Autodesk Inventor part; units mm, degrees
ref_plane "YZ Plane" through (0, 0, 0) normal (1, 0, 0) x (0, 1, 0)
ref_plane "XZ Plane" through (0, 0, 0) normal (0, 1, 0) x (-1, 0, 0)
ref_plane "XY Plane" through (0, 0, 0) normal (0, 0, 1) x (1, 0, 0)
sketch "Sketch1" plane through (0, 0, 0) normal (0, 1, 0) x (-1, 0, 0)
  line L0 (-690, -330) -> (690, -330)
  line L1 (690, -330) -> (690, 330)
  line L2 (690, 330) -> (-690, 330)
  line L3 (-690, 330) -> (-690, -330)
  line L4 (-690, -330) -> (690, 330) construction
  line L5 (690, -330) -> (-690, 330) construction
  point P0 (0, 0)
  dimension "d0" = 1380
  dimension "d1" = 660
extrude "Extrusion1" add sketch "Sketch1" along normal blind 60
sketch "Sketch2" plane through (0, 60, 0) normal (0, 1, 0) x (1, 0, 0)
  line L0 (-660, 300) -> (-360, 300) construction
  line L1 (-360, 300) -> (-360, -300) construction
  line L2 (-360, -300) -> (-660, -300) construction
  line L3 (-660, -300) -> (-660, 300) construction
  line L4 (-660, 300) -> (-360, -300) construction
  line L5 (-360, 300) -> (-660, -300) construction
  line L6 (-690, 330) -> (-690, -330)
  line L7 (-690, 0) -> (690, 0) construction
  line L8 (690, -330) -> (690, 330) construction
  line L9 (-370, 290) -> (-650, 290)
  line L10 (-650, 290) -> (-650, -290)
  line L11 (-650, -290) -> (-370, -290)
  line L12 (-370, -290) -> (-370, 290)
  line L13 (-20, 300) -> (-20, -300) construction
  line L14 (-30, -290) -> (-30, 290)
  line L15 (-30, 290) -> (-310, 290)
  line L16 (-320, 300) -> (-20, 300) construction
  line L17 (-310, 290) -> (-310, -290)
  line L18 (-320, -300) -> (-320, 300) construction
  line L19 (-320, 300) -> (-20, -300) construction
  line L20 (-20, 300) -> (-320, -300) construction
  line L21 (-310, -290) -> (-30, -290)
  line L22 (-20, -300) -> (-320, -300) construction
  line L23 (320, 300) -> (320, -300) construction
  line L24 (310, -290) -> (310, 290)
  line L25 (310, 290) -> (30, 290)
  line L26 (20, 300) -> (320, 300) construction
  line L27 (30, 290) -> (30, -290)
  line L28 (20, -300) -> (20, 300) construction
  line L29 (20, 300) -> (320, -300) construction
  line L30 (320, 300) -> (20, -300) construction
  line L31 (30, -290) -> (310, -290)
  line L32 (320, -300) -> (20, -300) construction
  line L33 (660, 300) -> (660, -300) construction
  line L34 (650, -290) -> (650, 290)
  line L35 (650, 290) -> (370, 290)
  line L36 (360, 300) -> (660, 300) construction
  line L37 (370, 290) -> (370, -290)
  line L38 (360, -300) -> (360, 300) construction
  line L39 (360, 300) -> (660, -300) construction
  line L40 (660, 300) -> (360, -300) construction
  line L41 (370, -290) -> (650, -290)
  line L42 (660, -300) -> (360, -300) construction
  point P0 (0, 0)
  point P1 (-510, 0)
  point P2 (-170, 0)
  point P3 (170, 0)
  point P4 (510, 0)
  dimension "d4" = 300
  dimension "d5" = 600
  dimension "d6" = 30
  dimension "d7" = 10
  dimension "d10" = 340
extrude "Extrusion2" add sketch "Sketch2" along normal blind 255
sketch "Sketch3" plane through (0, 315, 0) normal (0, 1, 0) x (1, 0, 0)
  line L0 (-650, 290) -> (-650, -290) construction
  line L1 (-650, -290) -> (-370, -290) construction
  line L2 (-370, -290) -> (-370, 290) construction
  line L3 (-370, 290) -> (-650, 290) construction
  line L4 (-30, 290) -> (-310, 290) construction
  line L5 (-310, 290) -> (-310, -290) construction
  line L6 (-310, -290) -> (-30, -290) construction
  line L7 (-30, -290) -> (-30, 290) construction
  line L8 (310, 290) -> (30, 290) construction
  line L9 (30, 290) -> (30, -290) construction
  line L10 (30, -290) -> (310, -290) construction
  line L11 (310, -290) -> (310, 290) construction
  line L12 (650, 290) -> (370, 290) construction
  line L13 (370, 290) -> (370, -290) construction
  line L14 (370, -290) -> (650, -290) construction
  line L15 (650, -290) -> (650, 290) construction
  line L16 (-360, 300) -> (-360, -300)
  line L17 (-360, -300) -> (-660, -300)
  line L18 (-660, -300) -> (-660, 300)
  line L19 (-660, 300) -> (-360, 300)
  line L20 (-20, 300) -> (-320, 300)
  line L21 (-320, 300) -> (-320, -300)
  line L22 (-320, -300) -> (-20, -300)
  line L23 (-20, -300) -> (-20, 300)
  line L24 (20, 300) -> (320, 300)
  line L25 (320, 300) -> (320, -300)
  line L26 (320, -300) -> (20, -300)
  line L27 (20, -300) -> (20, 300)
  line L28 (360, -300) -> (360, 300)
  line L29 (360, 300) -> (660, 300)
  line L30 (660, 300) -> (660, -300)
  line L31 (660, -300) -> (360, -300)
  point P0 (0, 0)
  dimension "d17" = 10
  dimension "d18" = 10
  dimension "d19" = 10
  dimension "d20" = 10
extrude "Extrusion3" add sketch "Sketch3" along normal blind 40
sketch "Sketch4" plane through (0, 0, 0) normal (0, -1, 0) x (1, 0, 0)
  circle A0 centre (-200, 0) radius 50
  circle A1 centre (200, 0) radius 50
  line L0 (-200, 0) -> (200, 0) construction
  point P0 (0, 0)
  point P1 (0, 0)
  dimension "d23" = 100
  dimension "d24" = 100
  dimension "d25" = 400
extrude "Extrusion4" cut sketch "Sketch4" against normal blind 80
properties part number "SACMI PH1500 30X60 DIE SET TILES BOTTOM MOLD"
Model file for the job. Use its own axes, mm. A direction names the side the tool comes from. Coordinates: 2 decimals unless noted, no trailing zeros. Write each loop counter-clockwise with the first axis right and the second up, starting at its lowest first coordinate (ties: lowest second). Pieces come first, ordered by that corner, then holes. Notation, with made-up numbers: (66.25, 81.25) - (92.25, 81.25) arc R14 cw to (92.25, 96.25) - close; hole circle Ø2 at (-12.5, 9.5). An arc over 180 degrees is marked (long way). Use a Markdown table: item, result. Add a question column.
Item 1: Drop flat-ended pins along their axis: pin 1 (20 mm diameter, centred on x = 126.5, y = 340.5, fed in from -Z); pin 2 (12 mm diameter, centred on y = 118, z = 125.5, fed in from +X); pin 3 (1.5 mm diameter, centred on x = 463.5, y = 132.5, fed in from -Z). Give the stop position or say it passes through.
Item 2: Drill centre lines: line 1 along X through (y, z) = (233.5, -58.5); line 2 along Z through (x, y) = (200, 45); line 3 along Z through (x, y) = (-503.5, 103.5). Where is each one in solid material? Low to high.
Item 3: 3-axis set-ups, long thin cutter, end or side, ignore diameter. For faces 1 (the face through (512, 335, 300)), 2 (the face through (-168, 186, -290)), 3 (the face through (150.05, 39.44, 2.2)), 4 (the face through (508, 186, 290)): which of +Z, -Z, +X, -X, +Y, -Y reach the whole face in a straight line?
Item 4: Band-saw the part on A-A, the plane y = 166. Write the cut outline in (x, z).
Item 5: Band-saw the part on C-C, the plane x = -200. Write the cut outline in (y, z), and give its area (4 significant figures).
Item 6: Band-saw the part on B-B, the plane x = -391. Write the cut outline in (y, z).
Item 7: Two-plate mould, pull along Y, no slides. Class faces 5 (the face through (660, 335, -4)), 6 (the face through (168, 355, -4)), 7 (the face through (-172, 186, 290)): pulls with the +Y half, pulls with the -Y half, needs draft (parallel to the pull), parting line crosses it, or undercut.
Item 8: Band-saw the part on D-D, the plane x = 231.5. Write the cut outline in (y, z), and give its area (3 significant figures).
A:
| question | item | result |
|---|---|---|
| 1 | pin 1 | stops at z = -300 |
| 1 | pin 2 | stops at x = 650 |
| 1 | pin 3 | stops at z = -290 |
| 2 | line 1 | x = -650 to -370, -310 to -30, 30 to 310, 370 to 650 |
| 2 | line 2 | z = -330 to -50, 50 to 330 |
| 2 | line 3 | z = -290 to 290 |
| 3 | face 1 | +Z, +X, -X, +Y |
| 3 | face 2 | -Z, +X, -X |
| 3 | face 3 | -Y |
| 3 | face 4 | +Z, +X, -X |
| 4 | outline | (-650, -290) - (-370, -290) - (-370, 290) - (-650, 290) - close; (-310, -290) - (-30, -290) - (-30, 290) - (-310, 290) - close; (30, -290) - (310, -290) - (310, 290) - (30, 290) - close; (370, -290) - (650, -290) - (650, 290) - (370, 290) - close |
| 5 | outline | (0, -330) - (60, -330) - (60, -290) - (315, -290) - (315, -300) - (355, -300) - (355, 300) - (315, 300) - (315, 290) - (60, 290) - (60, 330) - (0, 330) - (0, 50) - (80, 50) - (80, -50) - (0, -50) - close |
| 5 | area | 203,500 mm² |
| 6 | outline | (0, -330) - (60, -330) - (60, -290) - (315, -290) - (315, -300) - (355, -300) - (355, 300) - (315, 300) - (315, 290) - (60, 290) - (60, 330) - (0, 330) - close |
| 7 | face 5 | needs draft |
| 7 | face 6 | pulls with the +Y half |
| 7 | face 7 | undercut |
| 8 | outline | (0, -330) - (60, -330) - (60, -290) - (315, -290) - (315, -300) - (355, -300) - (355, 300) - (315, 300) - (315, 290) - (60, 290) - (60, 330) - (0, 330) - (0, 38.83) - (80, 38.83) - (80, -38.83) - (0, -38.83) - close |
| 8 | area | 205,000 mm² |
